Part model, mm, in its own coordinate system. A direction names the side the tool comes from. Give positions to 0.01 mm unless a question says otherwise; leave off trailing zeros. Write each loop counter-clockwise with the first axis right and the second up, starting at its lowest first coordinate (ties: lowest second). Pieces come first, ordered by that corner, then holes. Notation, with made-up numbers: M 38,81 L 55,81 A26 ccw 55,120 Z; hole C -18.5,-4.75 d4. An arc over 180 degrees is marked long. Answer as CSV lines item,"result". Start each with the question number.
Item 1: Two-plate mould, pull along Y, no slides. Class faces 3 (the flat face through (-55, 25, 9)), 4 (the cylindrical face through (-17.5, 15.83, 30.44)), 5 (the flat face through (-38, 50, 23)), 6 (the flat face through (-22, 0, 30)): +Y half, -Y half, draft (parallel to the pull), parting line (faces both ways), or undercut.
Item 2: Band-saw the part on A-A, the plane z = 23.5. List the corners of the cut face in (x, y).
Item 3: 3-axis set-ups, long thin cutter, end or side, ignore diameter. For faces 1 (the flat face through (-20, 42, 30)), 2 (the flat face through (-40, 31, 39)): which of +Z, -Z, +X, -X, +Y, -Y reach the whole face in a straight line?
Item 4: Band-saw the part on C-C, the plane x = -45. List the corners of the cut face in (y, z).
Item 5: Pin check, flat tips, straight feed: pin 1 (5 mm diameter, centred on x = -11, z = 42.5, fed in from +Y); pin 2 (5 mm diameter, centred on y = 17.5, z = 50.5, fed in from -X); pin 3 (10 mm diameter, centred on y = 31.5, z = 7.5, fed in from +X); pin 4 (12 mm diameter, centred on x = -42.5, y = 24.5, fed in from +Z). Stop position of each tip, or through.
Item 6: Band-saw the part on B-B, the plane z = 52. List the corners of the cut face in (x, y), then the cut area to 3 significant figures.
Item 7: Band-saw the part on D-D, the plane z = 37. List the corners of the cut face in (x, y), then the cut area to 3 significant figures.
Item 8: Wall check: L1, parallel to Z at x = -48.5, y = 4; L2, parallel to Y at x = -34, z = 35; L3, parallel to X at y = 6, z = 45.5. Give the ranges that are in metal, low to high. Write a range as from..to.
from build123d import *

# Parameters (mm, degrees)
SKETCH1_W           = 15
SKETCH1_H           = 50
BOSS_EXTRUDE1_DEPTH = 18
BOSS_EXTRUDE2_DEPTH = 60
SKETCH2_R           = 10
CUT_EXTRUDE2_DEPTH  = 60


with BuildPart() as part:
    # Sketch1 → Boss-Extrude1 (new body)
    with BuildSketch(Plane.XY):
        with Locations((-47.5, 25)):
            Rectangle(SKETCH1_W, SKETCH1_H)
    extrude(amount=BOSS_EXTRUDE1_DEPTH)

    # Sketch1_3 → Boss-Extrude2 (add)
    with BuildSketch(Plane.XY):
        Polygon((0, 22), (-28, 50), (-40, 50), (-40, 0), (0, 0), align=None)
    extrude(amount=BOSS_EXTRUDE2_DEPTH)

    # Sketch2 → Cut-Extrude2 (cut)
    with BuildSketch(Plane(origin=(11, 11, 0), x_dir=(0, 0, -1), z_dir=(0.7071067811865464, 0.7071067811865488, 0))):
        with Locations(Location((-30, 33.556349186, 0), (0, 0, 90))):
            Circle(SKETCH2_R)
    extrude(amount=-CUT_EXTRUDE2_DEPTH, mode=Mode.SUBTRACT)


solid = part.part
Output:
1,face 3,"draft"
1,face 4,"undercut"
1,face 5,"+Y half"
1,face 6,"-Y half"
2,outline,"M -40,18.2 L -18.1,40.1 L -28,50 L -40,50 Z; M -36.71,0 L 0,0 L 0,22 L -7.35,29.35 Z"
3,face 1,"+Z, -Z, +X, +Y"
3,face 2,"+Z, -X, +Y, -Y"
4,outline,"M 0,0 L 50,0 L 50,18 L 0,18 Z"
5,pin 1,"y = 35.5"
5,pin 2,"x = -40"
5,pin 3,"x = -4.5"
5,pin 4,"z = 60"
6,outline,"M -40,0 L 0,0 L 0,22 L -28,50 L -40,50 Z"
6,area,"1,610 mm²"
7,outline,"M -40,17.56 L -17.78,39.78 L -28,50 L -40,50 Z; M -37.36,0 L 0,0 L 0,22 L -7.68,29.68 Z"
7,area,"1,060 mm²"
8,L1,"0..18"
8,L2,"0..1.21, 25.7..50"
8,L3,"-40..0"
